from build123d import *

# Parameters (mm, degrees)
BOX406008008_W     = 10
BOX406008008_H     = 10
BOX406008008_DEPTH = 19
CYLINDER079_R      = 1.75
CYLINDER079_DEPTH  = 17
BOX406008009_W     = 8
BOX406008009_H     = 8
BOX406008009_DEPTH = 11
CHAMFER004_SIZE    = 2
CHAMFER008_SIZE    = 0.5


with BuildPart() as cube343:
    # Box406008008 → Box406008008 (new body)
    with BuildSketch(Plane(origin=(-5, 1.1, 1.5), x_dir=(1, 0, 0), z_dir=(0, 0, 1))):
        with Locations((5, 5)):
            Rectangle(BOX406008008_W, BOX406008008_H)
    extrude(amount=BOX406008008_DEPTH)


with BuildPart() as motor_shaft_hole:
    # Cylinder079 → Cylinder079 (new body)
    with BuildSketch(Plane.XY.offset(9)):
        Circle(CYLINDER079_R)
    extrude(amount=CYLINDER079_DEPTH)

    # Cut064: cut Cube343
    add(cube343.part, mode=Mode.SUBTRACT)


with BuildPart() as chamfer008:
    # Box406008009 → Box406008009 (new body)
    with BuildSketch(Plane(origin=(-4, -4, 7), x_dir=(1, 0, 0), z_dir=(0, 0, 1))):
        with Locations((4, 4)):
            Rectangle(BOX406008009_W, BOX406008009_H)
    extrude(amount=BOX406008009_DEPTH)

    # Cut065: cut Motor Shaft Hole
    add(motor_shaft_hole.part, mode=Mode.SUBTRACT)

    # Chamfer004
    chamfer004_edges = [chamfer008.edges().sort_by_distance(p)[0] for p in [
        (-4, 0, 7),
        (0, -4, 7),
        (0, 4, 7),
        (4, 0, 7),
    ]]
    chamfer(chamfer004_edges, length=CHAMFER004_SIZE)

    # Chamfer008
    chamfer008_edges = [chamfer008.edges().sort_by_distance(p)[0] for p in [
        (1.649904, 0.583367, 18),
        (0, 1.1, 18),
        (-0.583367, -1.649904, 18),
    ]]
    chamfer(chamfer008_edges, length=CHAMFER008_SIZE)


solid = chamfer008.part
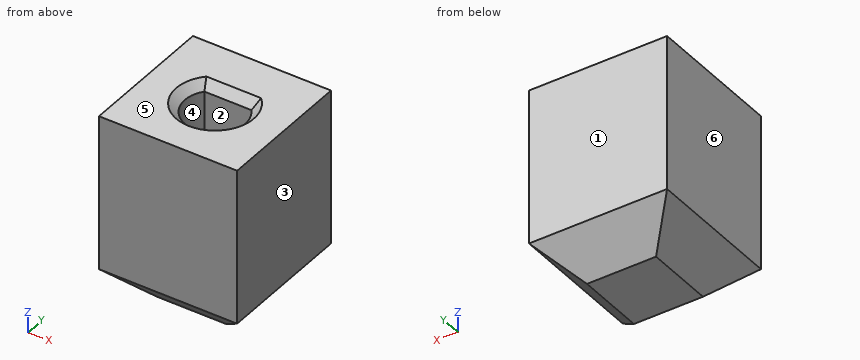
Design review of the part built by this model. Coordinates are the model's own, in mm. Face numbers are marked on the shaded views. A direction names the side the tool comes from. Give positions to 0.01 mm unless a question says otherwise; leave off trailing zeros. Write each loop counter-clockwise with the first axis right and the second up, starting at its lowest first coordinate (ties: lowest second). Pieces come first, ordered by that corner, then holes. Notation, with made-up numbers: M 85,-29 L 112,-29 A20 cw 112,2 Z; hole C 34,-16 d11. An arc over 180 degrees is marked long. Return JSON: item names as keys, results as strings. Group by question number.
Item 1: Take a section at A-A (z = 12). Give the boundary of the cut face in (x, y).
Item 2: Take a section at C-C (y = 0). Give the boundary of the cut face in (x, z), plus the area to 4 significant figures.
Item 3: Wall thickness on line 1 along X through (y, z) = (0, 12.5); line 2 along Y through (x, z) = (0, 11.5); line 3 along Z through (x, y) = (0, -0.25): over which ranges is each line inside the solid? List them lowest first.
Item 4: Take a section at D-D (x = 0). Give the boundary of the cut face in (y, z).
Item 5: Clearance check with flat-ended pins moving along their axes: pin 1 Ø1.4 at (x, y) = (0.5, 0) entering from +Z; pin 2 Ø4 at (x, y) = (0, 0) entering from +Z; pin 3 Ø1.5 at (x, y) = (1, 3) entering from -Z. State where each tip first meets the part, or that it passes through.
Item 6: Tool access review of the marked faces 1 and 2: name each direction out of +Z, -Z, +X, -X, +Y, -Y from which nothing blocks a thin tool from reaching the whole face with its end or side.
Item 7: The part is to be moulded in two halves that separate along X. For the marked faces 3, 4, 5 and 6, say which applies: pulls with the +X half, pulls with the -X half, needs draft (parallel to the pull), parting line crosses it, or undercut.
Item 8: Take a section at B-B (x = -2.75). Give the boundary of the cut face in (y, z).
Return value:
{
 "1": {"outline": "M -4,-4 L 4,-4 L 4,4 L -4,4 Z; hole M -1.36,1.1 A1.75 ccw long 1.36,1.1 Z"},
 "2": {"outline": "M -4,9 L -2,7 L 2,7 L 4,9 L 4,18 L 2.25,18 L 1.75,17.5 L 1.75,9 L -1.75,9 L -1.75,17.5 L -2.25,18 L -4,18 Z", "area": "52.25 mm2"},
 "3": {"line 1": "x = -4 to -1.75, 1.75 to 4", "line 2": "y = -4 to -1.75, 1.1 to 4", "line 3": "z = 7 to 9"},
 "4": {"outline": "M -4,9 L -2,7 L 2,7 L 4,9 L 4,18 L 1.6,18 L 1.1,17.5 L 1.1,9 L -1.75,9 L -1.75,17.5 L -2.25,18 L -4,18 Z"},
 "5": {"pin 1": "stops at z = 9", "pin 2": "stops at z = 18", "pin 3": "stops at z = 7.25"},
 "6": {"face 1": "+Z, -Z, +X, -X, +Y", "face 2": "+Z"},
 "7": {"face 3": "pulls with the +X half", "face 4": "undercut", "face 5": "needs draft", "face 6": "pulls with the -X half"},
 "8": {"outline": "M -4,9 L -2.75,7.75 L 2.75,7.75 L 4,9 L 4,18 L -4,18 Z"}
}
